```python
from build123d import *

# Parameters (mm, degrees)
SKETCH_1_W      = 23
SKETCH_1_H      = 12
EXTRUDE_1_DEPTH = 16.3
SKETCH_2_W      = 32.5
SKETCH_2_H      = 12
SKETCH_2_R      = 1.1
EXTRUDE_2_DEPTH = 2.5
SKETCH_3_W      = 23
SKETCH_3_H      = 12
EXTRUDE_3_DEPTH = 4.4
EXTRUDE_4_DEPTH = 4.1
SKETCH_5_R      = 2.4
EXTRUDE_5_DEPTH = 3.3


with BuildPart() as part:
    # 草图1 → 凸台-拉伸1 (new body)
    with BuildSketch(Plane.XY):
        Rectangle(SKETCH_1_W, SKETCH_1_H)
    extrude(amount=EXTRUDE_1_DEPTH)

    # 草图2 → 凸台-拉伸2 (add)
    with BuildSketch(Plane.XY.offset(16.3)):
        Rectangle(SKETCH_2_W, SKETCH_2_H)
        with Locations((-13.9, 0)):
            Circle(SKETCH_2_R, mode=Mode.SUBTRACT)
        with Locations((13.9, 0)):
            Circle(SKETCH_2_R, mode=Mode.SUBTRACT)
    extrude(amount=EXTRUDE_2_DEPTH)

    # 草图3 → 凸台-拉伸3 (add)
    with BuildSketch(Plane.XY.offset(18.8)):
        Rectangle(SKETCH_3_W, SKETCH_3_H)
    extrude(amount=EXTRUDE_3_DEPTH)

    # 草图4 → 凸台-拉伸4 (add)
    with BuildSketch(Plane.XY.offset(23.2)):
        with BuildLine():
            ThreePointArc((0.049982862, 2.279844344), (-11.5, 0), (0.049982862, -2.279844344))
            ThreePointArc((0.049982862, -2.279844344), (3.575804369, 0), (0.049982862, 2.279844344))
        make_face()
    extrude(amount=EXTRUDE_4_DEPTH)

    # 草图5 → 凸台-拉伸5 (add)
    with BuildSketch(Plane.XY.offset(27.3)):
        with Locations((-5.5, 0)):
            Circle(SKETCH_5_R)
    extrude(amount=EXTRUDE_5_DEPTH)


solid = part.part
```
For this review, take the finished solid that the model builds, in its own axes (mm). A direction names the side the tool comes from. Coordinates: 2 decimals unless noted, no trailing zeros. Write each loop counter-clockwise with the first axis right and the second up, starting at its lowest first coordinate (ties: lowest second). Pieces come first, ordered by that corner, then holes.
(1) Add section B-B on y = -4. Give the boundary of the cut face in (x, z), then the cut area to 3 significant figures.
(2) Tool access review of faces 1 (the face through (-10, -5, 23.2)), 2 (the face through (11.5, 0, 8)), 3 (the face through (-13.9, 1.4, 16.3)), 4 (the face through (-2, 0, 27.3)), 5 (the face through (13.8, 1.4, 18.8)): name each direction out of +Z, -Z, +X, -X, +Y, -Y from which nothing blocks a thin tool from reaching the whole face with its end or side.
(3) Wall thickness on probe 1 along Y at (x, z) = (-13.9, 17.9); probe 2 along X at (y, z) = (-5, 19); probe 3 along Z at (x, y) = (-11, -2.25): over which ranges is each line inside the solid? List them lowest first.
(4) For pin 1 Ø5 at (y, z) = (3.5, 6.5) entering from -X; pin 2 Ø3.5 at (x, y) = (-13.9, 0) entering from +Z; pin 3 Ø3 at (x, y) = (13.9, 0) entering from -Z, all flat-tipped, find the tip position at first contact; note any pin that passes through.
(5) Add section D-D on z = 5. Give the boundary of the cut face in (x, y), then the cut area to 3 significant figures.
(6) Add section C-C on x = 12. Give the boundary of the cut face in (y, z), then the cut area to 3 significant figures.
(7) Add section A-A on x = -13.9. Give the boundary of the cut face in (y, z), then the cut area to 3 significant figures.
Answer sheet:
1. outline: (-16.25, 16.3) - (-11.5, 16.3) - (-11.5, 0) - (11.5, 0) - (11.5, 16.3) - (16.25, 16.3) - (16.25, 18.8) - (11.5, 18.8) - (11.5, 23.2) - (-1.03, 23.2) - (-1.03, 27.3) - (-9.97, 27.3) - (-9.97, 23.2) - (-11.5, 23.2) - (-11.5, 18.8) - (-16.25, 18.8) - close
1. area: 594 mm2
2. face 1: +Z, -X, -Y
2. face 2: -Z, +X, +Y, -Y
2. face 3: -Z, -X, +Y, -Y
2. face 4: +Z
2. face 5: +Z, +X, +Y, -Y
3. probe 1: y = -6 to -1.1, 1.1 to 6
3. probe 2: x = -11.5 to 11.5
3. probe 3: z = 0 to 27.3
4. pin 1: stops at x = -11.5
4. pin 2: stops at z = 18.8
4. pin 3: stops at z = 16.3
5. outline: (-11.5, -6) - (11.5, -6) - (11.5, 6) - (-11.5, 6) - close
5. area: 276 mm2
6. outline: (-6, 16.3) - (6, 16.3) - (6, 18.8) - (-6, 18.8) - close
6. area: 30.0 mm2
7. outline: (-6, 16.3) - (-1.1, 16.3) - (-1.1, 18.8) - (-6, 18.8) - close; (1.1, 16.3) - (6, 16.3) - (6, 18.8) - (1.1, 18.8) - close
7. area: 24.5 mm2
